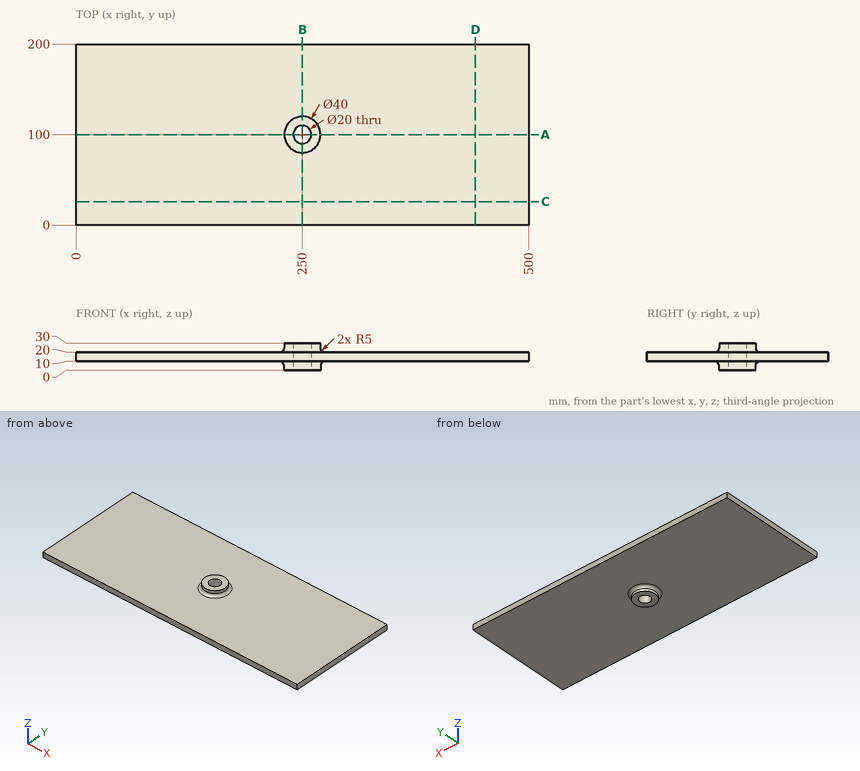
Source: three-view drawing plus pictorial views. Frame: mm from the lowest corner of the part. Round coordinates to 2 decimals unless told otherwise and drop trailing zeros. Loops run counter-clockwise (first coordinate to the right, second up) from the corner with the lowest first, then second, coordinate; pieces in that order, holes last. Notation, with made-up numbers: (26, -17.75) -> (57, -17.75) arc R14 ccw to (57, -3.75) -> close; hole circle Ø2 at (58, 0). An arc over 180 degrees is marked (long way). Use one line per item in the form item = value.
Item 1: Cut plane C-C on y = 26. Output: boundary loops of the cut face in (x, z), then the cut area to 3 significant figures.
Evaluation:
outline = (0, 10) -> (500, 10) -> (500, 20) -> (0, 20) -> close
area = 5,000 mm2
Item 2: Material intervals for probe 1 along Y at (x, z) = (250, 15.25); probe 2 along X at (y, z) = (91.5, 7); probe 3 along Z at (x, y) = (323, 9), sorted ascending.
Evaluation:
probe_1 = 0 to 90, 110 to 200
probe_2 = 231.44 to 244.73, 255.27 to 268.56
probe_3 = 10 to 20
Item 3: Cut plane B-B on x = 250. Output: boundary loops of the cut face in (y, z).
Evaluation:
outline = (0, 10) -> (75, 10) arc R5 cw to (80, 5) -> (80, 0) -> (90, 0) -> (90, 30) -> (80, 30) -> (80, 25) arc R5 cw to (75, 20) -> (0, 20) -> close; (110, 0) -> (120, 0) -> (120, 5) arc R5 cw to (125, 10) -> (200, 10) -> (200, 20) -> (125, 20) arc R5 cw to (120, 25) -> (120, 30) -> (110, 30) -> close
Item 4: Cut plane D-D on x = 441. Output: boundary loops of the cut face in (y, z).
Evaluation:
outline = (0, 10) -> (200, 10) -> (200, 20) -> (0, 20) -> close
Item 5: Cut plane A-A on y = 100. Output: boundary loops of the cut face in (x, z), then the cut area to 3 significant figures.
Evaluation:
outline = (0, 10) -> (225, 10) arc R5 cw to (230, 5) -> (230, 0) -> (240, 0) -> (240, 30) -> (230, 30) -> (230, 25) arc R5 cw to (225, 20) -> (0, 20) -> close; (260, 0) -> (270, 0) -> (270, 5) arc R5 cw to (275, 10) -> (500, 10) -> (500, 20) -> (275, 20) arc R5 cw to (270, 25) -> (270, 30) -> (260, 30) -> close
area = 5,220 mm2
Item 6: Contact query for flat-ended pins moving along their axis: pin 1 Ø4 at (x, y) = (425, 112) entering from -Z; pin 2 Ø18 at (x, y) = (250, 100) entering from +Z; pin 3 Ø5 at (x, y) = (351.5, 135.5) entering from +Z. Output: stop coordinate, or through.
Evaluation:
pin_1 = 10
pin_2 = through
pin_3 = 20
